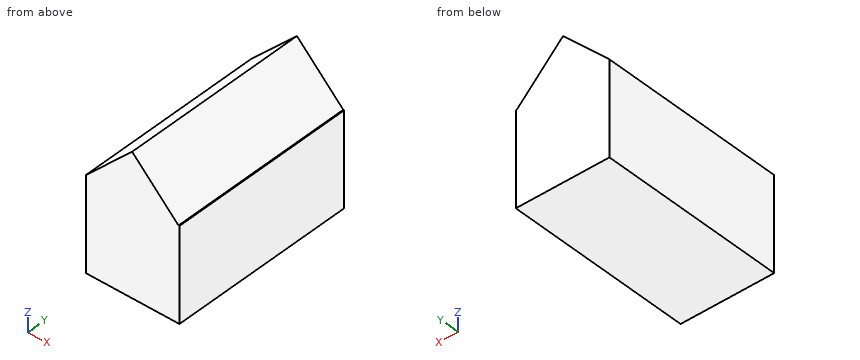
```python
from build123d import *

# Parameters (mm, degrees)
BOX001_W               = 7
BOX001_H               = 20
BOX001_DEPTH           = 7
BOX001_PLACEMENT_ANGLE = 45
BOX_W                  = 10
BOX_H                  = 20
BOX_DEPTH              = 10


with BuildPart() as cub001:
    # Box001 → Box001 (new body)
    with BuildSketch(Plane.XY):
        with Locations((3.5, 10)):
            Rectangle(BOX001_W, BOX001_H)
    extrude(amount=BOX001_DEPTH)


with BuildPart() as cub001_1:
    # Box001 placement: moved
    add(cub001.part.moved(Location((0, 0, 10))).rotate(Axis((0, 0, 10), (0, 1, 0)), BOX001_PLACEMENT_ANGLE))


with BuildPart() as fusion:
    # Box → Box (new body)
    with BuildSketch(Plane.XY):
        with Locations((5, 10)):
            Rectangle(BOX_W, BOX_H)
    extrude(amount=BOX_DEPTH)

    # Fusion: union Cub001
    add(cub001_1.part)


with BuildPart() as fusion_1:
    # Fusion placement: moved
    add(fusion.part.moved(Location((-4, -10, 0))))


solid = fusion_1.part
```
Geometry: final body of the model. Coordinates: model frame, mm. Round coordinates to 2 decimals unless told otherwise and drop trailing zeros. Order: outer loops, then holes, each group sorted by start corner. A loop starts at its lowest first (then second) coordinate and runs counter-clockwise, first axis right, second up. Notation, with made-up numbers: (-27.75, 82.5) -> (10.25, 82.5) arc R20 ccw to (10.25, 93.5) -> close; hole circle Ø3 at (-8.75, 83.25). An arc over 180 degrees is marked (long way). Write each question's results on one line, items separated by ' | '.
Q1. Section query C-C (z = 10.75). Output: boundary loops of the cut face in (x, y), and give its area (3 significant figures).
Response values:
outline: (-3.25, -10) -> (5.15, -10) -> (5.15, 10) -> (-3.25, 10) -> close | area: 168 mm²
Q2. Section query B-B (x = 5.25). Output: boundary loops of the cut face in (y, z).
Response values:
outline: (-10, 0) -> (10, 0) -> (10, 10.65) -> (-10, 10.65) -> close
Q3. Section query A-A (y = -2). Output: boundary loops of the cut face in (x, z).
Response values:
outline: (-4, 0) -> (6, 0) -> (6, 10) -> (5.9, 10) -> (0.95, 14.95) -> (-4, 10) -> close
Q4. Pin query (flat end, axial travel): pin 1 Ø3 at (x, y) = (-2.5, 7.5) entering from +Z; pin 2 Ø5 at (y, z) = (-7, 13) entering from -X. Return the tip coordinate at first contact, or that it passes through.
Response values:
pin 1: z = 13 | pin 2: x = -3.5
Q5. Ray query, line 1 along Z through (x, y) = (1, 4.5); line 2 along X through (y, z) = (8, 13.25); line 3 along Z through (x, y) = (1.25, -1.25). Return the intervals inside material, ascending.
Response values:
line 1: 0 to 14.9 | line 2: -0.75 to 2.65 | line 3: 0 to 14.65
